Source: CAD feature listing. Evaluate the final solid. Frame: model axes, mm. Round coordinates to 2 decimals unless told otherwise and drop trailing zeros. Write each loop counter-clockwise with the first axis right and the second up, starting at its lowest first coordinate (ties: lowest second). Pieces come first, ordered by that corner, then holes. Notation, with made-up numbers: M 26,40 L 58,40 A21 cw 58,60 Z; hole C -25.5,-37.5 d6. An arc over 180 degrees is marked long. Answer in a Markdown table with one row per item. Add a question column.
Item 1: Contact query for flat-ended pins moving along their axis: pin 1 (2 mm diameter, centred on x = 10, y = -24.5, fed in from +Z); pin 2 (6 mm diameter, centred on y = -5, z = -252, fed in from +X); pin 3 (1 mm diameter, centred on x = -19, y = -29, fed in from +Z). Output: stop coordinate, or through.
Item 2: Cut plane A-A on x = 20. Return loops of the section in (y, z) (3 decimals).
Item 3: Material intervals for probe 1 along Z at (x, y) = (-5, -21.5); probe 2 along X at (y, z) = (-3.5, 129.5); probe 3 along X at (y, z) = (-11.5, -152), sorted ascending.
Item 4: Cut plane D-D on z = 98. Return loops of the section in (x, y), and give its area (3 significant figures).
Item 5: Cut plane B-B on y = -26. Return loops of the section in (x, z).
Item 6: Cut plane C-C on x = -18.5. Return loops of the section in (y, z), and give its area (3 significant figures).
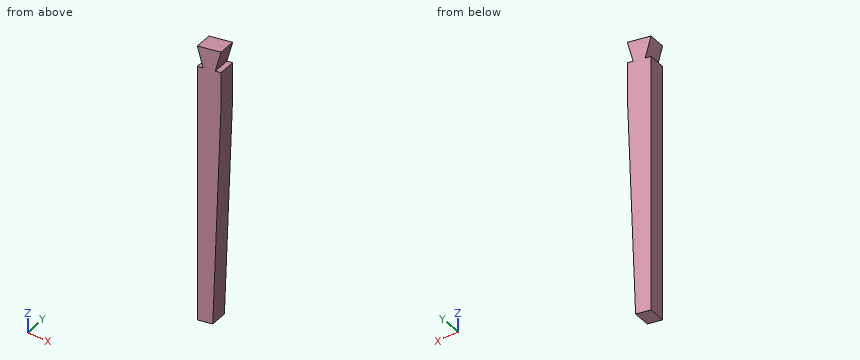
from build123d import *

# Parameters (mm, degrees)
F1_DEPTH = 33.782
F3_DEPTH = 33.783
F5_DEPTH = 33.783


with BuildPart() as f1:
    # F0 (on Front) → F1 (new body)
    with BuildSketch(Plane.XZ):
        Polygon((25.4, -304.8), (25.4, 304.8), (-25.4, 294.216667), (-25.4, -315.383333), align=None)
    extrude(amount=F1_DEPTH)

    # F2 (on face) → F3 (cut, through all)
    with BuildSketch(Plane.XZ.offset(33.782)):
        Polygon((25.4, 184.15), (7.671917, -308.493351), (25.4, -304.8), align=None)
    extrude(amount=-F3_DEPTH, mode=Mode.SUBTRACT)

    # F4 (on face) → F5 (cut, through all)
    with BuildSketch(Plane.XZ.offset(33.782)):
        Polygon((-25.4, 294.216667), (-25.4, 248.812286), (-12.966949, 251.402505), align=None)
        Polygon((25.4, 259.395619), (25.4, 304.8), (12.966949, 256.8054), align=None)
    extrude(amount=-F5_DEPTH, mode=Mode.SUBTRACT)


solid = f1.part
Results below:
| question | item | result |
|---|---|---|
| 1 | pin 1 | z = 301.8 |
| 1 | pin 2 | x = 9.81 |
| 1 | pin 3 | z = 295.65 |
| 2 | outline | M -33.782,34.09 L 0,34.09 L 0,258.271 L -33.782,258.271 Z; M -33.782,283.955 L 0,283.955 L 0,303.675 L -33.782,303.675 Z |
| 3 | probe 1 | -311.13 to 298.47 |
| 3 | probe 2 | -25.4 to 23.43 |
| 3 | probe 3 | -25.4 to 13.3 |
| 4 | outline | M -25.4,-33.78 L 22.3,-33.78 L 22.3,0 L -25.4,0 Z |
| 4 | area | 1,610 mm2 |
| 5 | outline | M -25.4,-315.38 L 7.67,-308.49 L 25.4,184.15 L 25.4,259.4 L 12.97,256.81 L 25.4,304.8 L -25.4,294.22 L -12.97,251.4 L -25.4,248.81 Z |
| 6 | outline | M -33.78,-313.95 L 0,-313.95 L 0,250.25 L -33.78,250.25 Z; M -33.78,270.46 L 0,270.46 L 0,295.65 L -33.78,295.65 Z |
| 6 | area | 19,900 mm2 |
